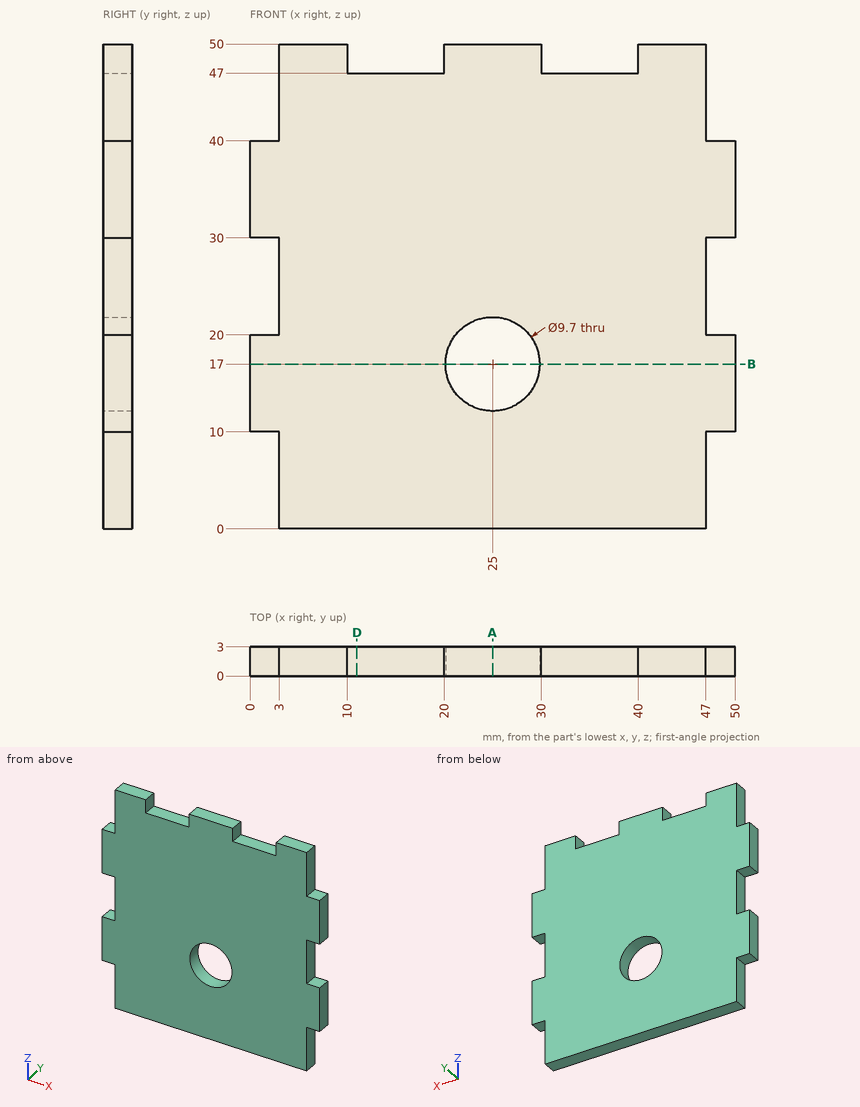
Source: three-view drawing plus pictorial views. Frame: mm from the lowest corner of the part. Give positions to 0.01 mm unless a question says otherwise; leave off trailing zeros. Order: outer loops, then holes, each group sorted by start corner. A loop starts at its lowest first (then second) coordinate and runs counter-clockwise, first axis right, second up. Notation, with made-up numbers: (-25.75, 18.25) -> (-4.75, 18.25) arc R21 ccw to (-4.75, 33.25) -> close; hole circle Ø11 at (10.5, -33.5). An arc over 180 degrees is marked (long way). Put each result on its own line as item: value.
Q1. Section B-B, the plane z = 17. Return loops of the section in (x, y).
Here are the results:
outline: (0, 0) -> (20.15, 0) -> (20.15, 3) -> (0, 3) -> close; (29.85, 0) -> (50, 0) -> (50, 3) -> (29.85, 3) -> close
Q2. Pin query (flat end, axial travel): pin 1 (1.5 mm diameter, centred on x = 48, y = 2, fed in from -Z); pin 2 (1.5 mm diameter, centred on y = 1.5, z = 43.5, fed in from +X); pin 3 (1.5 mm diameter, centred on x = 37, y = 1, fed in from +Z). Return the tip coordinate at first contact, or that it passes through.
Here are the results:
pin 1: stops at z = 10
pin 2: stops at x = 47
pin 3: stops at z = 47
Q3. Section A-A, the plane x = 25. Return loops of the section in (y, z), then the cut area to 3 significant figures.
Here are the results:
outline: (0, 0) -> (3, 0) -> (3, 12.15) -> (0, 12.15) -> close; (0, 21.85) -> (3, 21.85) -> (3, 50) -> (0, 50) -> close
area: 121 mm^2
Q4. Material intervals for L1, parallel to X at y = 0.95, z = 17; L2, parallel to Z at x = 47.5, y = 2.85; L3, parallel to Z at x = 31.5, y = 2.35, sorted ascending.
Here are the results:
L1: x = 0 to 20.15, 29.85 to 50
L2: z = 10 to 20, 30 to 40
L3: z = 0 to 47
Q5. Section D-D, the plane x = 11. Return loops of the section in (y, z).
Here are the results:
outline: (0, 0) -> (3, 0) -> (3, 47) -> (0, 47) -> close
